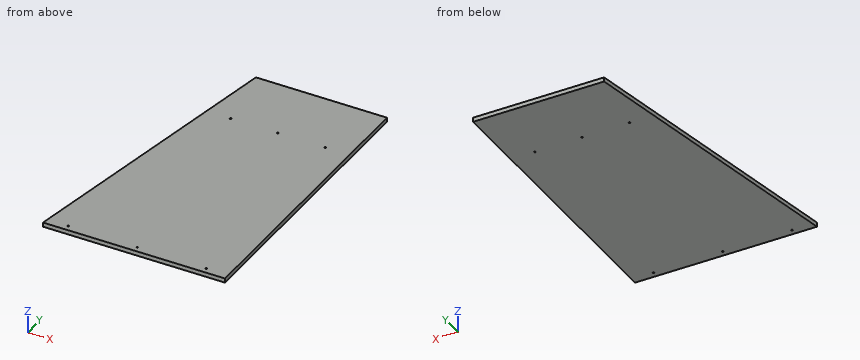
from build123d import *

# Parameters (mm, degrees)
SKETCH_1_R      = 1.1
EXTRUDE_1_DEPTH = 6


with BuildPart() as part:
    # Эскиз1 → Бобышка-Вытянуть1 (new body)
    with BuildSketch(Plane.XY):
        Polygon((0, 0), (69.841269841, 400), (250, 400), (250, 0), align=None)
        with Locations((86.803174603, 307)):
            Circle(SKETCH_1_R, mode=Mode.SUBTRACT)
        with Locations((151.803174603, 307)):
            Circle(SKETCH_1_R, mode=Mode.SUBTRACT)
        with Locations((30, 8)):
            Circle(SKETCH_1_R, mode=Mode.SUBTRACT)
        with Locations((220, 8)):
            Circle(SKETCH_1_R, mode=Mode.SUBTRACT)
        with Locations((125, 8)):
            Circle(SKETCH_1_R, mode=Mode.SUBTRACT)
        with Locations((216.803174603, 307)):
            Circle(SKETCH_1_R, mode=Mode.SUBTRACT)
    extrude(amount=EXTRUDE_1_DEPTH)


solid = part.part
Geometry: final body of the model. Coordinates: model frame, mm. Coordinates: 2 decimals unless noted, no trailing zeros. Order: outer loops, then holes, each group sorted by start corner. A loop starts at its lowest first (then second) coordinate and runs counter-clockwise, first axis right, second up.
(1) Material intervals for probe 1 along Y at (x, z) = (220, 3.3); probe 2 along X at (y, z) = (68, 1.6); probe 3 along X at (y, z) = (262, 3.65), sorted ascending.
(2) Section query A-A (z = 3.7). Return the cut outline in (x, y).
(3) First-contact query: pin 1 (1.8 mm diameter, centred on x = 216.8, y = 307, fed in from -Z). Flat tip, straight axial feed; report the tip coordinate or a pass-through.
(4) Section query B-B (x = 41.5). Return the cut outline in (y, z).
(5) Section query C-C (y = 100). Return the cut outline in (x, z), plus the area to 3 significant figures.
Solution:
1. probe 1: y = 0 to 6.9, 9.1 to 400
1. probe 2: x = 11.87 to 250
1. probe 3: x = 45.75 to 250
2. outline: (0, 0) - (250, 0) - (250, 400) - (69.84, 400) - close; hole circle Ø2.2 at (30, 8); hole circle Ø2.2 at (86.8, 307); hole circle Ø2.2 at (125, 8); hole circle Ø2.2 at (151.8, 307); hole circle Ø2.2 at (216.8, 307); hole circle Ø2.2 at (220, 8)
3. pin 1: passes through
4. outline: (0, 0) - (237.68, 0) - (237.68, 6) - (0, 6) - close
5. outline: (17.46, 0) - (250, 0) - (250, 6) - (17.46, 6) - close
5. area: 1,400 mm2
